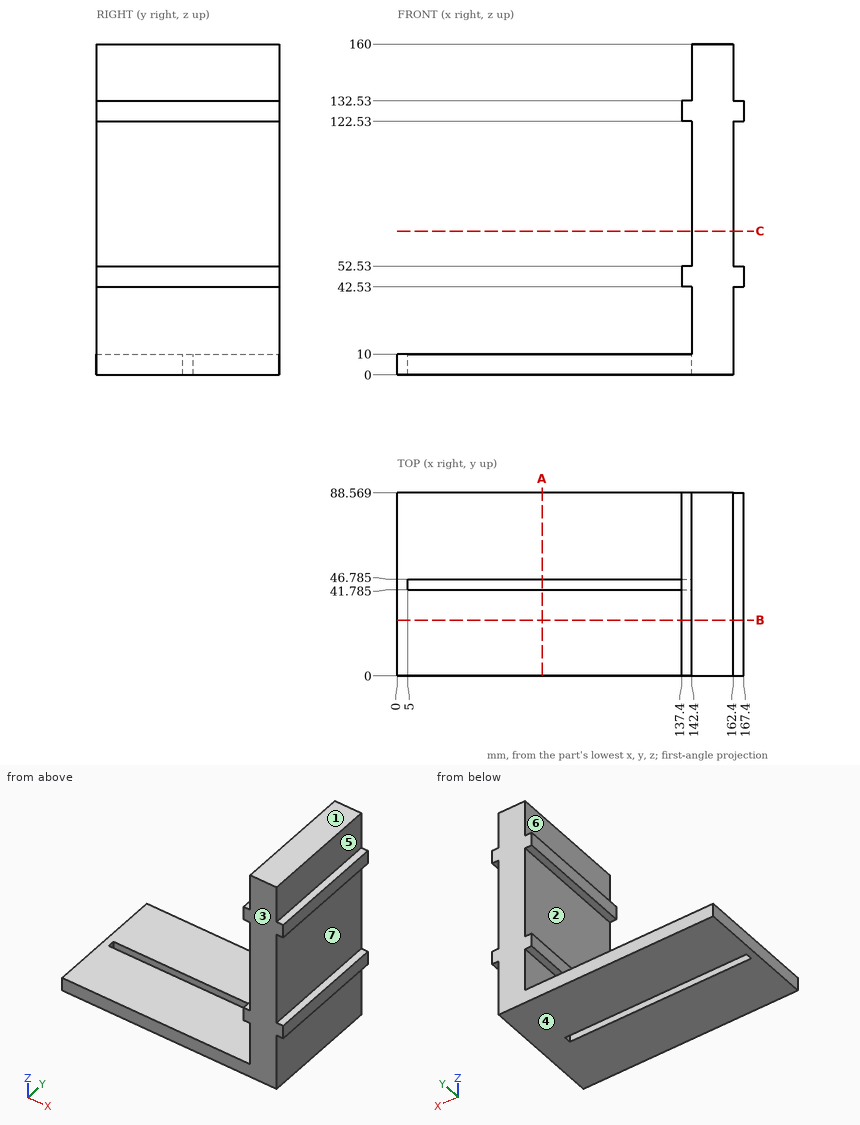
For this review, use the dimensioned drawing (mm, ordinates from the lowest corner) and the shaded views. A direction names the side the tool comes from. Coordinates: 2 decimals unless noted, no trailing zeros. Write each loop counter-clockwise with the first axis right and the second up, starting at its lowest first coordinate (ties: lowest second). Pieces come first, ordered by that corner, then holes. Notation, with made-up numbers: (20, 77.25) - (26, 77.25) arc R24 ccw to (26, 93.25) - close; hole circle Ø10 at (-29.75, 82.5). An arc over 180 degrees is marked (long way). Answer in a Markdown table with one row per item. Add a question column.
Q1. Consider section C-C on z = 69.5. Give the boundary of the cut face in (x, y), then the cut area to 3 significant figures.
Q2. Consider section B-B on y = 27. Give the boundary of the cut face in (x, z).
Q3. Clearance check with flat-ended pins moving along their axes: pin 1 (6 mm diameter, centred on x = 74.5, y = 26.5, fed in from +Z); pin 2 (4 mm diameter, centred on y = 44.5, z = 6.5, fed in from +X); pin 3 (2.5 mm diameter, centred on x = 164, y = 44.5, fed in from +Z); pin 4 (11 mm diameter, centred on x = 87, z = 5, fed in from -Y). State where each tip first meets the part, or that it passes through.
Q4. Draft analysis for pull direction Z (two halves, no side actions). For the marked faces 1, 2, 3 and 4, state which applies: +Z half, -Z half, draft (parallel to the pull), parting line (faces both ways), or undercut.
Q5. Consider section A-A on x = 70. Give the boundary of the cut face in (y, z) (1 decimal).
Q6. For the marked faces 5, 6 and 7, list the 3-axis set-ups (+Z, -Z, +X, -X, +Y, -Y) from which the entire face can be reached by the end or side of a thin tool; tool diameter is ignored.
Q7. To check wall thickness, follow line 1 along Z through (x, y) = (140, 13); line 2 along X through (y, z) = (81.5, 134); line 3 along Z through (x, y) = (99, 15.5). State the ranges of each line that lie inside material, in increasing order. Write a range as from..to.
Answers below:
| question | item | result |
|---|---|---|
| 1 | outline | (142.4, 0) - (162.4, 0) - (162.4, 88.57) - (142.4, 88.57) - close |
| 1 | area | 1,770 mm² |
| 2 | outline | (0, 0) - (162.4, 0) - (162.4, 42.53) - (167.4, 42.53) - (167.4, 52.53) - (162.4, 52.53) - (162.4, 122.53) - (167.4, 122.53) - (167.4, 132.53) - (162.4, 132.53) - (162.4, 160) - (142.4, 160) - (142.4, 132.53) - (137.4, 132.53) - (137.4, 122.53) - (142.4, 122.53) - (142.4, 52.53) - (137.4, 52.53) - (137.4, 42.53) - (142.4, 42.53) - (142.4, 10) - (0, 10) - close |
| 3 | pin 1 | z = 10 |
| 3 | pin 2 | x = 162.4 |
| 3 | pin 3 | z = 132.53 |
| 3 | pin 4 | y = 0 |
| 4 | face 1 | +Z half |
| 4 | face 2 | undercut |
| 4 | face 3 | draft |
| 4 | face 4 | -Z half |
| 5 | outline | (0, 0) - (41.8, 0) - (41.8, 10) - (0, 10) - close; (46.8, 0) - (88.6, 0) - (88.6, 10) - (46.8, 10) - close |
| 6 | face 5 | +Z, +X, +Y, -Y |
| 6 | face 6 | +Z, -X, +Y, -Y |
| 6 | face 7 | +X, +Y, -Y |
| 7 | line 1 | 0..10, 42.53..52.53, 122.53..132.53 |
| 7 | line 2 | 142.4..162.4 |
| 7 | line 3 | 0..10 |
